from build123d import *

# Parameters (mm, degrees)
SKETCH_W        = 230
SKETCH_H        = 140
PAD_DEPTH       = 40
SKETCH001_W     = 222
SKETCH001_H     = 132
POCKET_DEPTH    = 34
SKETCH002_W     = 98
SKETCH002_H     = 40
SKETCH002_W_2   = 12
SKETCH002_H_2   = 12
POCKET001_DEPTH = 6.001
SKETCH004_R     = 6
SKETCH004_W     = 14
SKETCH004_H     = 14
POCKET002_DEPTH = 4
SKETCH003_W     = 14
SKETCH003_H     = 6
POCKET003_DEPTH = 4
SKETCH005_R     = 2.5
SKETCH005_R_2   = 1
PAD001_DEPTH    = 5


with BuildPart() as part:
    # Sketch → Pad (new body)
    with BuildSketch(Plane.XY):
        with Locations((115, 70)):
            Rectangle(SKETCH_W, SKETCH_H)
    extrude(amount=PAD_DEPTH)

    # Sketch001 (on Face6 of Pad) → Pocket (cut)
    with BuildSketch(Plane.XY.offset(40)):
        with Locations((115, 70)):
            Rectangle(SKETCH001_W, SKETCH001_H)
    extrude(amount=-POCKET_DEPTH, mode=Mode.SUBTRACT)

    # Sketch002 (on Face11 of Pocket) → Pocket001 (cut, through all)
    with BuildSketch(Plane.XY.offset(6)):
        with Locations((171, 100)):
            Rectangle(SKETCH002_W, SKETCH002_H)
        with Locations((180, 59)):
            Rectangle(SKETCH002_W_2, SKETCH002_H_2)
        with Locations((197, 59)):
            Rectangle(SKETCH002_W_2, SKETCH002_H_2)
        with Locations((214, 59)):
            Rectangle(SKETCH002_W_2, SKETCH002_H_2)
    extrude(amount=-POCKET001_DEPTH, mode=Mode.SUBTRACT)

    # Sketch004 (on Face1 of Pocket001) → Pocket002 (cut)
    with BuildSketch(Plane.XZ):
        with Locations((20, 20)):
            Circle(SKETCH004_R)
        with Locations((149, 17)):
            Rectangle(SKETCH004_W, SKETCH004_H)
    extrude(amount=-POCKET002_DEPTH, mode=Mode.SUBTRACT)

    # Sketch003 (on Face3 of Pocket001) → Pocket003 (cut)
    with BuildSketch(Plane.YZ.offset(230)):
        with Locations((24, 12)):
            Rectangle(SKETCH003_W, SKETCH003_H)
    extrude(amount=-POCKET003_DEPTH, mode=Mode.SUBTRACT)

    # Sketch005 (on Face32 of Pocket002) → Pad001 (join)
    with BuildSketch(Plane.XY.offset(6)):
        with Locations((217.5, 127.5)):
            Circle(SKETCH005_R)
        with Locations((217.5, 127.5)):
            Circle(SKETCH005_R_2, mode=Mode.SUBTRACT)
        with Locations((124.5, 127.5)):
            Circle(SKETCH005_R)
        with Locations((124.5, 127.5)):
            Circle(SKETCH005_R_2, mode=Mode.SUBTRACT)
        with Locations((217.5, 72.5)):
            Circle(SKETCH005_R)
        with Locations((217.5, 72.5)):
            Circle(SKETCH005_R_2, mode=Mode.SUBTRACT)
        with Locations((124.5, 72.5)):
            Circle(SKETCH005_R)
        with Locations((124.5, 72.5)):
            Circle(SKETCH005_R_2, mode=Mode.SUBTRACT)
        with Locations((114.5, 127.5)):
            Circle(SKETCH005_R)
        with Locations((114.5, 127.5)):
            Circle(SKETCH005_R_2, mode=Mode.SUBTRACT)
        with Locations((114.5, 72.5)):
            Circle(SKETCH005_R)
        with Locations((114.5, 72.5)):
            Circle(SKETCH005_R_2, mode=Mode.SUBTRACT)
        with Locations((49.5, 127.8)):
            Circle(SKETCH005_R)
        with Locations((49.5, 127.8)):
            Circle(SKETCH005_R_2, mode=Mode.SUBTRACT)
        with Locations((49.5, 72.8)):
            Circle(SKETCH005_R)
        with Locations((49.5, 72.8)):
            Circle(SKETCH005_R_2, mode=Mode.SUBTRACT)
        with Locations((175.5, 35.5)):
            Circle(SKETCH005_R)
        with Locations((175.5, 35.5)):
            Circle(SKETCH005_R_2, mode=Mode.SUBTRACT)
        with Locations((175.5, 12.5)):
            Circle(SKETCH005_R)
        with Locations((175.5, 12.5)):
            Circle(SKETCH005_R_2, mode=Mode.SUBTRACT)
        with Locations((215, 24)):
            Circle(SKETCH005_R)
        with Locations((195, 24)):
            Circle(SKETCH005_R)
        with Locations((161.5, 7.5)):
            Circle(SKETCH005_R)
        with Locations((161.5, 7.5)):
            Circle(SKETCH005_R_2, mode=Mode.SUBTRACT)
        with Locations((135.5, 7.5)):
            Circle(SKETCH005_R)
        with Locations((135.5, 7.5)):
            Circle(SKETCH005_R_2, mode=Mode.SUBTRACT)
        with Locations((135.5, 43.5)):
            Circle(SKETCH005_R)
        with Locations((135.5, 43.5)):
            Circle(SKETCH005_R_2, mode=Mode.SUBTRACT)
        with Locations((161.5, 43.5)):
            Circle(SKETCH005_R)
        with Locations((161.5, 43.5)):
            Circle(SKETCH005_R_2, mode=Mode.SUBTRACT)
    extrude(amount=PAD001_DEPTH)


solid = part.part
Geometry: final body of the model. Coordinates: model frame, mm. A direction names the side the tool comes from. Coordinates: 2 decimals unless noted, no trailing zeros. Loops run counter-clockwise (first coordinate to the right, second up) from the corner with the lowest first, then second, coordinate; pieces in that order, holes last. Notation, with made-up numbers: (-31.5, 39.25) - (-3.5, 39.25) arc R13 ccw to (-3.5, 58.25) - close; hole circle Ø10 at (-19.75, -33.5). An arc over 180 degrees is marked (long way). One line per question, with ' | ' between items. Start each with the question number.
(1) Cut plane B-B on y = 24. Output: boundary loops of the cut face in (x, z).
(2) Cut plane D-D on x = 79. Output: boundary loops of the cut face in (y, z).
(3) First-contact query: pin 1 (4 mm diameter, centred on x = 124, y = 128.5, fed in from +Z); pin 2 (1.6 mm diameter, centred on x = 49.5, y = 72.8, fed in from +Z). Flat tips, straight axial feed; report the tip coordinate or a pass-through.
(4) Reachability of faces 3 (the flat face through (195, 24, 11)), 4 (the flat face through (197, 65, 3)), 5 (the cylindrical face through (126.885, 73.251, 8.465)) from +Z, -Z, +X, -X, +Y, -Y: full face, straight path, thin tool, end or side. Return the list, or none.
(5) Ray query, L1, parallel to Y at x = 69, z = 22; L2, parallel to X at y = 47, z = 19.5; L3, parallel to Y at x = 49.5, z = 7.5. Return the intervals inside material, ascending. Write a range as from..to.
(6) Cut plane A-A on x = 181. Output: boundary loops of the cut face in (y, z).
(7) Draft query along Y for faces 1 (the flat face through (80, 3, 40)), 2 (the flat face through (220, 100, 3)). Return one class per face: +Y half, -Y half, draft (parallel to the pull), parting line (faces both ways), or undercut.
(8) Cut plane C-C on z = 20. Output: boundary loops of the cut face in (x, y).
Here are the results:
1) outline: (0, 0) - (230, 0) - (230, 9) - (226, 9) - (226, 6) - (217.5, 6) - (217.5, 11) - (212.5, 11) - (212.5, 6) - (197.5, 6) - (197.5, 11) - (192.5, 11) - (192.5, 6) - (4, 6) - (4, 40) - (0, 40) - close; (226, 15) - (230, 15) - (230, 40) - (226, 40) - close
2) outline: (0, 0) - (140, 0) - (140, 40) - (136, 40) - (136, 6) - (4, 6) - (4, 40) - (0, 40) - close
3) pin 1: z = 11 | pin 2: z = 6
4) face 3: +Z, +X | face 4: +Z, -Z | face 5: +Z
5) L1: 0..4, 136..140 | L2: 0..4, 226..230 | L3: 0..4, 70.3..71.8, 73.8..75.3, 125.3..126.8, 128.8..130.3, 136..140
6) outline: (0, 0) - (53, 0) - (53, 6) - (4, 6) - (4, 40) - (0, 40) - close; (65, 0) - (80, 0) - (80, 6) - (65, 6) - close; (120, 0) - (140, 0) - (140, 40) - (136, 40) - (136, 6) - (120, 6) - close
7) face 1: draft | face 2: undercut
8) outline: (0, 0) - (14, 0) - (14, 4) - (4, 4) - (4, 136) - (226, 136) - (226, 4) - (156, 4) - (156, 0) - (230, 0) - (230, 140) - (0, 140) - close; (26, 0) - (142, 0) - (142, 4) - (26, 4) - close
